from build123d import *

# Parameters (mm, degrees)
SKETCH1_R           = 10
BOSS_EXTRUDE1_DEPTH = 4.5
SKETCH2_R           = 3
BOSS_EXTRUDE2_DEPTH = 21.5
SKETCH3_R           = 2
CUT_EXTRUDE1_DEPTH  = 6.5
SKETCH4_R           = 1.6
CUT_EXTRUDE2_DEPTH  = 27
SKETCH5_R           = 2.85
CUT_EXTRUDE3_DEPTH  = 3.2


with BuildPart() as part:
    # Sketch1 → Boss-Extrude1 (new body)
    with BuildSketch(Plane.XY):
        Circle(SKETCH1_R)
    extrude(amount=BOSS_EXTRUDE1_DEPTH)

    # Sketch2 → Boss-Extrude2 (add)
    with BuildSketch(Plane.XY.offset(4.5)):
        Circle(SKETCH2_R)
    extrude(amount=BOSS_EXTRUDE2_DEPTH)

    # Sketch3 → Cut-Extrude1 (cut)
    with BuildSketch(Plane(origin=(0, 0, 0), x_dir=(-1, 0, 0), z_dir=(0, 0, -1))):
        Circle(SKETCH3_R)
    extrude(amount=-CUT_EXTRUDE1_DEPTH, mode=Mode.SUBTRACT)

    # Sketch4 → Cut-Extrude2 (cut, through all)
    with BuildSketch(Plane(origin=(0, 0, 0), x_dir=(-1, 0, 0), z_dir=(0, 0, -1))):
        with Locations((0, 6)):
            Circle(SKETCH4_R)
        with Locations((6, 0)):
            Circle(SKETCH4_R)
        with Locations((0, -6)):
            Circle(SKETCH4_R)
        with Locations((-6, 0)):
            Circle(SKETCH4_R)
    extrude(amount=-CUT_EXTRUDE2_DEPTH, mode=Mode.SUBTRACT)

    # Sketch5 → Cut-Extrude3 (cut)
    with BuildSketch(Plane.XY.offset(4.5)):
        with Locations((0, 6)):
            Circle(SKETCH5_R)
        with Locations((6, 0)):
            Circle(SKETCH5_R)
        with Locations((0, -6)):
            Circle(SKETCH5_R)
        with Locations((-6, 0)):
            Circle(SKETCH5_R)
    extrude(amount=-CUT_EXTRUDE3_DEPTH, mode=Mode.SUBTRACT)


solid = part.part
Verification items for the finished model (mm, model axes). A direction names the side the tool comes from. Give positions to 0.01 mm unless a question says otherwise; leave off trailing zeros. Write each loop counter-clockwise with the first axis right and the second up, starting at its lowest first coordinate (ties: lowest second). Pieces come first, ordered by that corner, then holes.
(1) Material ranges on line 1 (Y direction, x = 0, z = 3.05); line 2 (Y direction, x = 0, z = 0.8); line 3 (Z direction, x = -9, y = -3), recorded low to high.
(2) Access from +Z, -Z, +X, -X, +Y, -Y to the whole of each face (thin tool, end or side, straight path). Record for faces 4 (the face through (-0.371, 8.826, 2.922)), 5 (the face through (0, -2, 3)), 6 (the face through (0.35, 4.44, 0.64)).
(3) Cross-section at A-A (y = -6). Enter the section's corners in (x, z).
(4) Gauge pin test, flat ends, axial feed: pin 1 (2.5 mm diameter, centred on x = 0, y = -6, fed in from -Z); pin 2 (3 mm diameter, centred on x = -1, y = 6, fed in from +Z); pin 3 (3 mm diameter, centred on x = 0, y = 0, fed in from -Z); pin 4 (1.5 mm diameter, centred on x = 0.5, z = 8.5, fed in from -Y). Record the tip position at first contact, or that the pin passes through.
(5) Cross-section at C-C (z = 2.75). Enter the section's corners in (x, y).
(6) Mould release check, pull along Y, two halves, no side actions. Record for faces 1 (the face through (8.633, -1.092, 2.922)), 2 (the face through (-2.17, -9.76, 2.22)), 3 (the face through (0, 0, 26)): +Y half, -Y half, draft (parallel to the pull), parting line (faces both ways), or undercut.
(7) Cross-section at B-B (x = 0). Enter the section's corners in (y, z).
Worked out:
1. line 1: y = -10 to -8.85, -3.15 to -2, 2 to 3.15, 8.85 to 10
1. line 2: y = -10 to -7.6, -4.4 to -2, 2 to 4.4, 7.6 to 10
1. line 3: z = 0 to 4.5
2. face 4: +Z
2. face 5: -Z
2. face 6: +Z, -Z
3. outline: (-8, 0) - (-1.6, 0) - (-1.6, 1.3) - (-2.85, 1.3) - (-2.85, 4.5) - (-8, 4.5) - close; (1.6, 0) - (8, 0) - (8, 4.5) - (2.85, 4.5) - (2.85, 1.3) - (1.6, 1.3) - close
4. pin 1: passes through
4. pin 2: stops at z = 1.3
4. pin 3: stops at z = 6.5
4. pin 4: stops at y = -3
5. outline: circle Ø20 at (0, 0); hole circle Ø5.7 at (-6, 0); hole circle Ø5.7 at (0, -6); hole circle Ø5.7 at (0, 6); hole circle Ø4 at (0, 0); hole circle Ø5.7 at (6, 0)
6. face 1: undercut
6. face 2: parting line
6. face 3: draft
7. outline: (-10, 0) - (-7.6, 0) - (-7.6, 1.3) - (-8.85, 1.3) - (-8.85, 4.5) - (-10, 4.5) - close; (-4.4, 0) - (-2, 0) - (-2, 6.5) - (2, 6.5) - (2, 0) - (4.4, 0) - (4.4, 1.3) - (3.15, 1.3) - (3.15, 4.5) - (3, 4.5) - (3, 26) - (-3, 26) - (-3, 4.5) - (-3.15, 4.5) - (-3.15, 1.3) - (-4.4, 1.3) - close; (7.6, 0) - (10, 0) - (10, 4.5) - (8.85, 4.5) - (8.85, 1.3) - (7.6, 1.3) - close
